Source: CAD feature listing. Evaluate the final solid. Frame: model axes, mm. Face numbers are marked on the shaded views. Coordinates: 2 decimals unless noted, no trailing zeros. Write each loop counter-clockwise with the first axis right and the second up, starting at its lowest first coordinate (ties: lowest second). Pieces come first, ordered by that corner, then holes. Notation, with made-up numbers: (1, 9) - (44, 9) arc R14 cw to (44, 18) - close; hole circle Ø8 at (57.25, 73). An arc over 180 degrees is marked (long way). One line per question, with ' | ' between items. Start each with the question number.
Q1. Cut plane B-B, the plane x = 0. Give the number of separate pieces and of enclosed holes in the cut face, plus the area to 3 significant figures.
Q2. Draft query along Y for the marked faces 1, 2, 3 and 4. Return one class per face: +Y half, -Y half, draft (parallel to the pull), parting line (faces both ways), or undercut.
Q3. Contact query for flat-ended pins moving along their axis: P1, Ø3, axis at y = -3.5, z = 2, coming from the +X side; P2, Ø3, axis at x = 4.5, z = 5.5, coming from the -Y side; P3, Ø1.4, axis at y = -4, z = 5, coming from the +X side. Output: stop coordinate, or through.
Q4. Cut plane A-A, the plane y = 32. Return loops of the section in (x, z), plus the area to 4 significant figures.
Q5. Line query: line 1 (Y direction, x = -20, z = 1.5); line 2 (Y direction, x = -2, z = 1); line 3 (Y direction, x = 18, z = 3.75). Output: solid intervals per line, ascending.
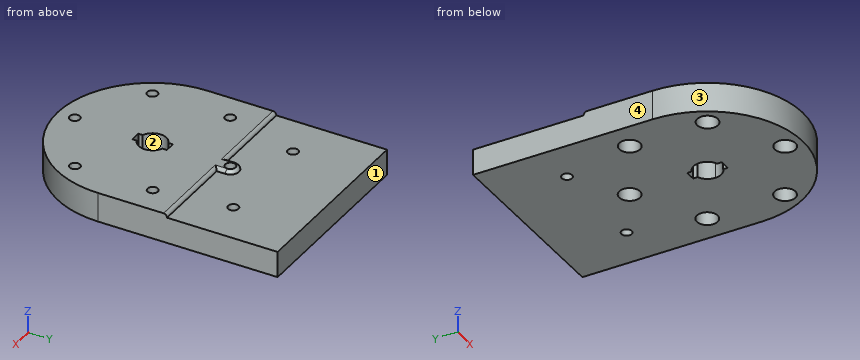
```python
from build123d import *

# Parameters (mm, degrees)
ESQUISSE1_W             = 100
ESQUISSE1_H             = 100.548113933
BOSS_EXTRU_1_DEPTH      = 8.5
ESQUISSE2_R             = 1.5
ENL_V_MAT_EXTRU_1_DEPTH = 73.637800077
ENL_V_MAT_EXTRU_6_DEPTH = 1
CONG_4_R                = 1
ESQUISSE4_R             = 3
ENL_V_MAT_EXTRU_7_DEPTH = 4


with BuildPart() as part:
    # Esquisse1 → Boss.-Extru.1 (new body)
    with BuildSketch(Plane.XY):
        with Locations((0, 1.725943033)):
            Rectangle(ESQUISSE1_W, ESQUISSE1_H)
        with BuildLine():
            Line((-1.5, 3.708099244), (-1.5, 5))
            Line((-1.5, 5), (1.5, 5))
            Line((1.5, 5), (1.5, 3.708099244))
            ThreePointArc((1.5, 3.708099244), (3.31662479, 2.236067977), (4, 0))
            ThreePointArc((4, 0), (3.31662479, -2.236067977), (1.5, -3.708099244))
            Line((1.5, -3.708099244), (1.5, -5))
            Line((1.5, -5), (-1.5, -5))
            Line((-1.5, -5), (-1.5, -3.708099244))
            ThreePointArc((-1.5, -3.708099244), (-4, 0), (-1.5, 3.708099244))
        make_face(mode=Mode.SUBTRACT)
    extrude(amount=BOSS_EXTRU_1_DEPTH)

    # Esquisse2 → Enlèv. mat.-Extru.1 (cut, through all)
    with BuildSketch(Plane.XY.offset(8.5)):
        with BuildLine():
            ThreePointArc((27.5, 0), (0, -27.5), (-27.5, 0))
            Line((-27.5, 0), (-27.5, 52))
            Line((-27.5, 52), (-50, 52))
            Line((-50, 52), (-50, -48.548113933))
            Line((-50, -48.548113933), (50, -48.548113933))
            Line((50, -48.548113933), (50, 52))
            Line((50, 52), (27.5, 52))
            Line((27.5, 52), (27.5, 0))
        make_face()
        with Locations((0, 22.5)):
            Circle(ESQUISSE2_R)
        with Locations((19.485571585, 11.25)):
            Circle(ESQUISSE2_R)
        with Locations((19.485571585, -11.25)):
            Circle(ESQUISSE2_R)
        with Locations((0, -22.5)):
            Circle(ESQUISSE2_R)
        with Locations((-19.485571585, -11.25)):
            Circle(ESQUISSE2_R)
        with Locations((-19.485571585, 11.25)):
            Circle(ESQUISSE2_R)
        with Locations((-15, 32)):
            Circle(ESQUISSE2_R)
        with Locations((15, 32)):
            Circle(ESQUISSE2_R)
    extrude(amount=-ENL_V_MAT_EXTRU_1_DEPTH, mode=Mode.SUBTRACT)

    # Esquisse3 → Enlèv. mat.-Extru.6 (cut)
    with BuildSketch(Plane.XY.offset(8.5)):
        with BuildLine():
            Line((27.5, 52), (-27.5, 52))
            Line((-27.5, 52), (-27.5, 20))
            Line((-27.5, 20), (-2.5, 20))
            Line((-2.5, 20), (-2.5, 22.5))
            ThreePointArc((-2.5, 22.5), (0, 25), (2.5, 22.5))
            Line((2.5, 22.5), (2.5, 20))
            Line((2.5, 20), (27.5, 20))
            Line((27.5, 20), (27.5, 52))
        make_face()
    extrude(amount=-ENL_V_MAT_EXTRU_6_DEPTH, mode=Mode.SUBTRACT)

    # Congé4
    cong_4_edges = [part.edges().sort_by_distance(p)[0] for p in [
        (-15, 20, 8.5),
        (15, 20, 8.5),
        (2.5, 21.25, 8.5),
        (-2.5, 21.25, 8.5),
        (0, 25, 8.5),
    ]]
    fillet(cong_4_edges, radius=CONG_4_R - 0.0001)  # a hair under: the kernel refuses the full size

    # Esquisse4 → Enlèv. mat.-Extru.7 (cut)
    with BuildSketch(Plane(origin=(0, 0, 0), x_dir=(-1, 0, 0), z_dir=(0, 0, -1))):
        with Locations((0, 22.5)):
            Circle(ESQUISSE4_R)
        with Locations((19.485571585, 11.25)):
            Circle(ESQUISSE4_R)
        with Locations((19.485571585, -11.25)):
            Circle(ESQUISSE4_R)
        with Locations((0, -22.5)):
            Circle(ESQUISSE4_R)
        with Locations((-19.485571585, -11.25)):
            Circle(ESQUISSE4_R)
        with Locations((-19.485571585, 11.25)):
            Circle(ESQUISSE4_R)
    extrude(amount=-ENL_V_MAT_EXTRU_7_DEPTH, mode=Mode.SUBTRACT)


solid = part.part
```
Reply:
1) separate pieces: 4 | enclosed holes: 0 | area: 489 mm^2
2) face 1: +Y half | face 2: undercut | face 3: -Y half | face 4: draft
3) P1: stops at x = 27.43 | P2: stops at y = -27.34 | P3: stops at x = 27.3
4) outline: (-27.5, 0) - (-16.5, 0) - (-16.5, 7.5) - (-27.5, 7.5) - close; (-13.5, 0) - (13.5, 0) - (13.5, 7.5) - (-13.5, 7.5) - close; (16.5, 0) - (27.5, 0) - (27.5, 7.5) - (16.5, 7.5) - close | area: 367.5 mm^2
5) line 1: y = -18.87 to -14.21, -8.29 to 8.29, 14.21 to 52 | line 2: y = -27.43 to -24.74, -20.26 to -3.46, 3.46 to 20.26, 24.74 to 52 | line 3: y = -20.79 to -13.86, -8.64 to 8.64, 13.86 to 52
